For this review, take the finished solid that the model builds, in its own axes (mm). Face numbers are marked on the shaded views. A direction names the side the tool comes from. Round coordinates to 2 decimals unless told otherwise and drop trailing zeros. Order: outer loops, then holes, each group sorted by start corner. A loop starts at its lowest first (then second) coordinate and runs counter-clockwise, first axis right, second up. Notation, with made-up numbers: (74.25, -1.75) - (91.25, -1.75) arc R17 ccw to (91.25, 27.25) - close; hole circle Ø11 at (46.5, 82.25). An arc over 180 degrees is marked (long way). One line per item, written item: value.
```python
from build123d import *
from build123d.topology import SkipClean

# Parameters (mm, degrees)
SKETCH1_R                   = 6.35
FLANGE_BOTTOM_DEPTH         = 7.9248
SKETCH2_R                   = 6.35
FLANGMIDBODY_DEPTH          = 3.175
FLANGELEGS_DEPTH            = 11.1252
FILLET1_R                   = 3.175
LOCKINGSHAFTHOLE_DEPTH      = 22.060567449
LOCKINGSHAFTHOLE_DEPTH_BACK = 22.060567449
SKETCH4_R                   = 0.635
FILLET3_R                   = 1.27
SKETCH5_R                   = 3.17246
CENTERSHAFTHOLE_DEPTH       = 24.970724451
SKETCH10_R                  = 0.889
SET_SCREW_DEPTH             = 22.060567449
SKETCH11_R                  = 0.889
SUB_DRILL_DEPTH             = 1.27


# Some blends are built 0.0001 mm under size
with BuildPart() as part:
    # Sketch1 → Flange Bottom (new body)
    with BuildSketch(Plane(origin=(-19.05, 0, 0), x_dir=(0, 0, -1), z_dir=(1, 0, 0))):
        Circle(SKETCH1_R)
    extrude(amount=FLANGE_BOTTOM_DEPTH)

    # Sketch2 → Flangmidbody (add)
    with BuildSketch(Plane(origin=(-11.1252, 0, 0), x_dir=(0, 0, -1), z_dir=(1, 0, 0))):
        Circle(SKETCH2_R)
    extrude(amount=FLANGMIDBODY_DEPTH)

    # Sketch3 → Flangelegs (add)
    with SkipClean():  # the faces are left unmerged after this step: merging them gives an invalid solid
        with BuildSketch(Plane(origin=(-7.9502, 0, 0), x_dir=(0, 0, -1), z_dir=(1, 0, 0))):
            with BuildLine():
                Line((-5.499261314, 3.175), (-3.965573729, 3.175))
                ThreePointArc((-3.965573729, 3.175), (-5.08, 0), (-3.965573729, -3.175))
                Line((-3.965573729, -3.175), (-5.499261314, -3.175))
                ThreePointArc((-5.499261314, -3.175), (-6.35, 0), (-5.499261314, 3.175))
            make_face()
            with BuildLine():
                Line((3.965573729, 3.175), (5.499261314, 3.175))
                ThreePointArc((5.499261314, 3.175), (6.35, 0), (5.499261314, -3.175))
                Line((5.499261314, -3.175), (3.965573729, -3.175))
                ThreePointArc((3.965573729, -3.175), (5.08, 0), (3.965573729, 3.175))
            make_face()
        extrude(amount=FLANGELEGS_DEPTH)

    # Fillet1
    fillet1_edges = [part.edges().sort_by_distance(p)[0] for p in [
        (3.175, -3.175, -4.732417522),
        (3.175, 3.175, -4.732417522),
        (3.175, -3.175, 4.732417522),
        (3.175, 3.175, 4.732417522),
    ]]
    fillet(fillet1_edges, radius=FILLET1_R - 0.0001)  # a hair under: the kernel refuses the full size

    # Sketch4 → Lockingshafthole (cut, two sides: drawn at the far end of the back side and taken through both)
    with BuildSketch(Plane.XY.offset(-LOCKINGSHAFTHOLE_DEPTH_BACK)):
        Circle(SKETCH4_R)
    extrude(amount=LOCKINGSHAFTHOLE_DEPTH + LOCKINGSHAFTHOLE_DEPTH_BACK, mode=Mode.SUBTRACT)

    # Fillet3
    # the kernel refuses this fillet: 1.27 mm, written as the material it adds along each edge
    with BuildSketch(Plane(origin=(-7.9502, 3.175, -0.790573729), x_dir=(1, 0, 0), z_dir=(0, 0, -1))) as fillet3_piece_1_section:
        with BuildLine():
            CenterArc((FILLET3_R, -FILLET3_R), FILLET3_R, 90, 90)
            Line((0, -FILLET3_R), (0, 0))
            Line((0, 0), (FILLET3_R, 0))
        make_face()
    fillet3_piece_1 = extrude(amount=7.883687585, mode=Mode.PRIVATE)
    fillet3_piece_1 = fillet3_piece_1 & Plane(origin=(-7.671308244, 0, 0), x_dir=(0, 0.4999999999999997, -0.8660254037844388), z_dir=(-1, 0, 0)) * Cylinder(6.35, 21, mode=Mode.PRIVATE)
    fillet3_piece_1 = fillet3_piece_1 - Plane(origin=(-7.671308244, 0, 0), x_dir=(0, -0.6249999999999998, -0.7806247497997999), z_dir=(-1, 0, 0)) * Cylinder(5.08, 21, mode=Mode.PRIVATE)
    add(fillet3_piece_1)
    with BuildSketch(Plane(origin=(-7.9502, -3.175, -8.674261314), x_dir=(1, 0, 0), z_dir=(0, 0, 1))) as fillet3_piece_2_section:
        with BuildLine():
            CenterArc((FILLET3_R, -FILLET3_R), FILLET3_R, 90, 90)
            Line((0, -FILLET3_R), (0, 0))
            Line((0, 0), (FILLET3_R, 0))
        make_face()
    fillet3_piece_2 = extrude(amount=7.883687585, mode=Mode.PRIVATE)
    fillet3_piece_2 = fillet3_piece_2 & Plane(origin=(-7.671308757, 0, 0), x_dir=(0, 0.4999999999999997, -0.8660254037844388), z_dir=(-1, 0, 0)) * Cylinder(6.35, 21, mode=Mode.PRIVATE)
    fillet3_piece_2 = fillet3_piece_2 - Plane(origin=(-7.671308757, 0, 0), x_dir=(0, -0.6249999999999998, -0.7806247497997999), z_dir=(-1, 0, 0)) * Cylinder(5.08, 21, mode=Mode.PRIVATE)
    add(fillet3_piece_2)
    with BuildSketch(Plane(origin=(-7.9502, -3.175, 0.790573729), x_dir=(0, -1, 0), z_dir=(0, 0, 1))) as fillet3_piece_3_section:
        with BuildLine():
            CenterArc((FILLET3_R, FILLET3_R), FILLET3_R, 180, 90)
            Line((0, FILLET3_R), (0, 0))
            Line((0, 0), (FILLET3_R, 0))
        make_face()
    fillet3_piece_3 = extrude(amount=7.883687585, mode=Mode.PRIVATE)
    fillet3_piece_3 = fillet3_piece_3 & Plane(origin=(-7.671308363, 0, 0), x_dir=(0, 0, -1), z_dir=(-1, 0, 0)) * Cylinder(6.35, 21, mode=Mode.PRIVATE)
    fillet3_piece_3 = fillet3_piece_3 - Plane(origin=(-7.671308363, 0, 0), x_dir=(0, 0.6250000000000004, 0.7806247497997995), z_dir=(-1, 0, 0)) * Cylinder(5.08, 21, mode=Mode.PRIVATE)
    add(fillet3_piece_3)
    with BuildSketch(Plane(origin=(-7.9502, 3.175, 8.674261314), x_dir=(0, 1, 0), z_dir=(0, 0, -1))) as fillet3_piece_4_section:
        with BuildLine():
            CenterArc((FILLET3_R, FILLET3_R), FILLET3_R, 180, 90)
            Line((0, FILLET3_R), (0, 0))
            Line((0, 0), (FILLET3_R, 0))
        make_face()
    fillet3_piece_4 = extrude(amount=7.883687585, mode=Mode.PRIVATE)
    fillet3_piece_4 = fillet3_piece_4 & Plane(origin=(-7.671308731, 0, 0), x_dir=(0, 0, -1), z_dir=(-1, 0, 0)) * Cylinder(6.35, 21, mode=Mode.PRIVATE)
    fillet3_piece_4 = fillet3_piece_4 - Plane(origin=(-7.671308731, 0, 0), x_dir=(0, 0.6250000000000004, 0.7806247497997995), z_dir=(-1, 0, 0)) * Cylinder(5.08, 21, mode=Mode.PRIVATE)
    add(fillet3_piece_4)

    # Sketch5 → CenterShaftHole (cut, through all)
    with BuildSketch(Plane.ZY.offset(19.05)):
        Circle(SKETCH5_R)
    extrude(amount=-CENTERSHAFTHOLE_DEPTH, mode=Mode.SUBTRACT)

    # Sketch10 → SET SCREW (cut, through all)
    with BuildSketch(Plane(origin=(0, 0, 0), x_dir=(1, 0, 0), z_dir=(0, 1, 0))):
        with Locations(Location((-15.24, 0, 0), (0, 0, 270))):
            Circle(SKETCH10_R)
    extrude(amount=-SET_SCREW_DEPTH, mode=Mode.SUBTRACT)

    # Sketch11 → SUB DRILL (cut)
    with BuildSketch(Plane.XY.offset(-6.35)):
        with Locations((-15.24, 0)):
            Circle(SKETCH11_R)
    extrude(amount=SUB_DRILL_DEPTH, mode=Mode.SUBTRACT)


solid = part.part
```
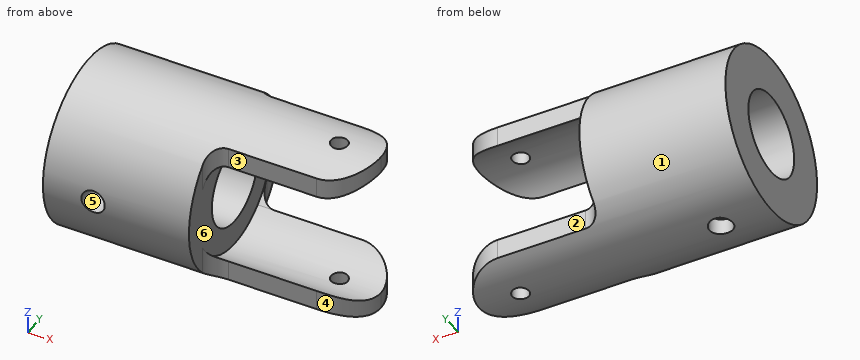
Item 1: For P1, Ø1, axis at x = 0, y = 3.5, coming from the +Z side; P2, Ø1.6, axis at x = -15.24, y = 0, coming from the -Z side; P3, Ø4, axis at y = -5, z = 1, coming from the +X side; P4, Ø1, axis at x = 0, y = 0, coming from the +Z side, all flat-tipped, find the tip position at first contact; note any pin that passes through.
Returned:
P1: z = 5.6
P2: z = -5.08
P3: x = -7.93
P4: through
Item 2: Take a section at C-C (y = -0.25). Write out the cut boundary in (x, z).
Returned:
outline: (-19.05, -6.35) - (-16.09, -6.35) - (-16.09, -5.08) - (-14.39, -5.08) - (-14.39, -6.35) - (-0.58, -6.35) - (-0.58, -5.07) - (-7.95, -5.07) - (-7.95, -3.16) - (-19.05, -3.16) - close; (-19.05, 3.16) - (-7.95, 3.16) - (-7.95, 5.07) - (-0.58, 5.07) - (-0.58, 6.35) - (-19.05, 6.35) - close; (0.58, -6.35) - (3.17, -6.35) - (3.17, -5.07) - (0.58, -5.07) - close; (0.58, 5.07) - (3.17, 5.07) - (3.17, 6.35) - (0.58, 6.35) - close
Item 3: Take a section at A-A (x = -5.5). Write out the cut boundary in (y, z) (3 decimals), plus the area to 3 significant figures.
Returned:
outline: (-3.175, -5.499) arc R6.35 ccw to (3.175, -5.499) - (3.175, -3.966) arc R5.08 cw to (-3.175, -3.966) - close; (-3.175, 3.966) arc R5.08 cw to (3.175, 3.966) - (3.175, 5.499) arc R6.35 ccw to (-3.175, 5.499) - close
area: 17.1 mm^2
Item 4: Take a section at B-B (z = 0). Write out the cut boundary in (x, y), plus the area to 3 significant figures.
Returned:
outline: (-19.05, -6.35) - (-16.13, -6.35) - (-16.13, -3.17) - (-19.05, -3.17) - close; (-19.05, 3.17) - (-7.95, 3.17) - (-7.95, 6.35) - (-19.05, 6.35) - close; (-14.35, -6.35) - (-7.95, -6.35) - (-7.95, -3.17) - (-14.35, -3.17) - close
area: 64.9 mm^2
Item 5: Take a section at D-D (x = -17). Write out the cut boundary in (y, z).
Returned:
outline: circle Ø12.7 at (0, 0); hole circle Ø6.34 at (0, 0)
Item 6: The part is to be moulded in two halves that separate along Y. For the marked faces 4, 5 and 6, say which applies: +Y half, -Y half, draft (parallel to the pull), parting line (faces both ways), or undercut.
Returned:
face 4: -Y half
face 5: draft
face 6: undercut
Item 7: Wall thickness on line 1 (X direction, y = -4.95, z = 0); line 2 (Z direction, x = -4.75, y = 0.25); line 3 (X direction, y = 5.25, z = -0.25): over which ranges is each line inside the solid? List them lowest first.
Returned:
line 1: -19.05 to -16.13, -14.35 to -7.95
line 2: -6.35 to -5.07, 5.07 to 6.35
line 3: -19.05 to -7.95
Item 8: Machinability: for the marked faces 1, 2 and 3, which of the approach directions +Z, -Z, +X, -X, +Y, -Y give a long, thin tool a straight path to every point of the face, cutting with its end or side? Answer none if there is none.
Returned:
face 1: +X, -X
face 2: +Z, -Z, +X, +Y
face 3: +Z, -Z, +X, -Y
